The drawing under review shows one solid part. Ordinate dimensions are in mm from its lowest x, y, z. A direction names the side the tool comes from. Round coordinates to 2 decimals unless told otherwise and drop trailing zeros. Order: outer loops, then holes, each group sorted by start corner. A loop starts at its lowest first (then second) coordinate and runs counter-clockwise, first axis right, second up.
1) Clearance check with flat-ended pins moving along their axes: P1, Ø12, axis at y = 34, z = 159, coming from the -X side; P2, Ø4, axis at y = 8, z = 226.5, coming from the +X side; P3, Ø2.5, axis at y = 8, z = 140, coming from the -X side. State where each tip first meets the part, or that it passes through.
2) To check wall thickness, follow L1, parallel to X at y = 99.5, z = 80; L2, parallel to Y at x = 46, z = 78 (1 decimal). State the ranges of each line that lie inside material, in increasing order.
3) Mouldability with a two-part tool opening along X and no side actions: class the marked faces 3, 4 and 5 as pulls with the +X half, pulls with the -X half, needs draft (parallel to the pull), parting line crosses it, or undercut.
4) Machinability: for the marked faces 1 and 2, which of the approach directions +Z, -Z, +X, -X, +Y, -Y give a long, thin tool a straight path to every point of the face, cutting with its end or side? Answer none if there is none.
5) Consider section A-A (x = 26). Give the boundary of the cut face in (y, z), then the cut area to 3 significant figures.
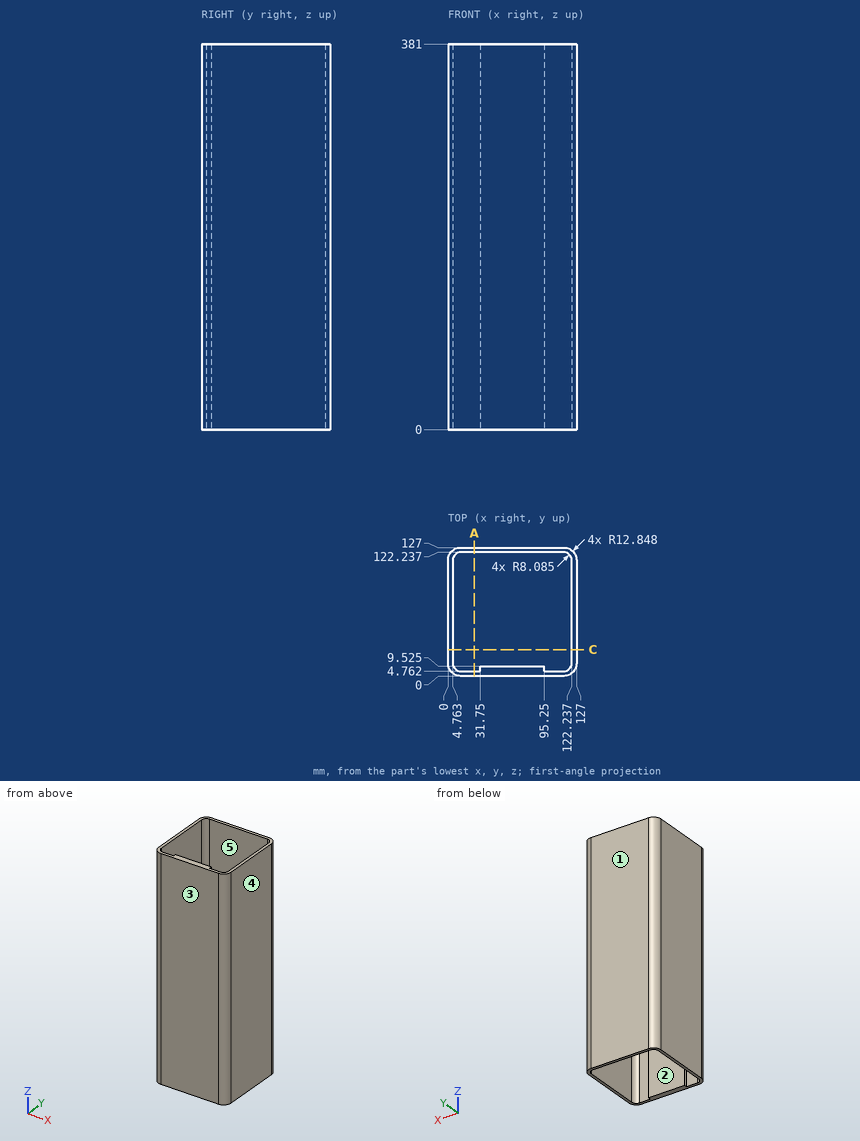
Answer below:
1. P1: stops at x = 0
1. P2: stops at x = 126.68
1. P3: stops at x = 0.51
2. L1: x = 0 to 4.76, 122.24 to 127
2. L2: y = 0 to 9.5, 122.2 to 127
3. face 3: needs draft
3. face 4: pulls with the +X half
3. face 5: undercut
4. face 1: +Z, -Z, +X, -X, +Y
4. face 2: +Z, -Z
5. outline: (0, 0) - (4.76, 0) - (4.76, 381) - (0, 381) - close; (122.24, 0) - (127, 0) - (127, 381) - (122.24, 381) - close
5. area: 3,630 mm2
